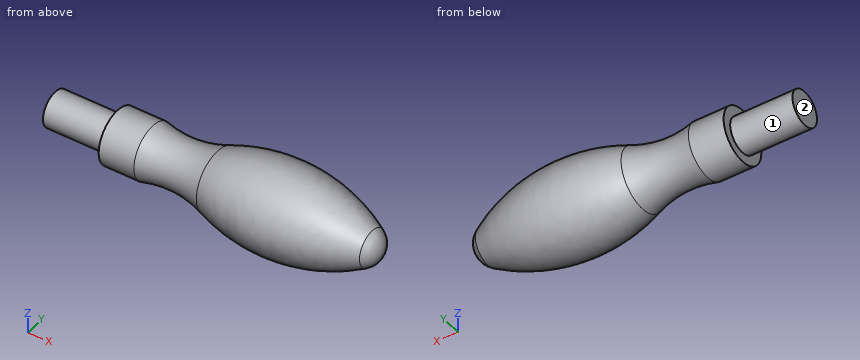
from build123d import *


with BuildPart() as f1:
    # F0 (on Front) → F1 (revolve)
    with BuildSketch(Plane.XZ):
        with BuildLine():
            Line((0, 6.5), (0, 0))
            Line((0, 0), (120.8, 0))
            ThreePointArc((120.8, 0), (119.780303, 3.855839), (116.987822, 6.703527))
            ThreePointArc((116.987822, 6.703527), (88.997191, 15.626515), (59.937706, 11.308939))
            ThreePointArc((59.937706, 11.308939), (48.07478, 8.717289), (36, 10))
            Line((36, 10), (23, 10))
            Line((23, 10), (23, 6.5))
            Line((23, 6.5), (0, 6.5))
        make_face()
    revolve(axis=Axis((60.4, 0, 0), (1, 0, 0)))


solid = f1.part
Read the model definition and answer for the solid it produces. Units are mm, in the model's axes. Face numbers are marked on the shaded views. A direction names the side the tool comes from. Coordinates: 2 decimals unless noted, no trailing zeros. Write each loop counter-clockwise with the first axis right and the second up, starting at its lowest first coordinate (ties: lowest second). Pieces come first, ordered by that corner, then holes. Notation, with made-up numbers: M 75.5,7.5 L 87.5,7.5 A19 ccw 87.5,30.5 Z; hole C -28,41 d2. An arc over 180 degrees is marked long. Use a Markdown table: item, result.
Q1. The part is cut by section A-A, the plane x = 29. Write down the section's boundary in (y, z).
Answer block:
| item | result |
|---|---|
| outline | C 0,0 d20 |
Q2. The part is cut by section B-B, the plane x = 42.5. Write down the section's boundary in (y, z), then the cut area to 3 significant figures.
Answer block:
| item | result |
|---|---|
| outline | C 0,0 d17.64 |
| area | 245 mm2 |
Q3. Which of the six approach directions +Z, -Z, +X, -X, +Y, -Y give full straight-line access (tool end or side, diameter ignored) to the marked faces 1 and 2?
Answer block:
| item | result |
|---|---|
| face 1 | -X |
| face 2 | +Z, -Z, -X, +Y, -Y |
Q4. Each of these flat-tipped pins is pushed along its axis until it touches: pin 1 Ø2 at (x, z) = (21, 4) entering from +Y; pin 2 Ø2 at (x, z) = (82.5, 5) entering from +Y; pin 3 Ø1 at (y, z) = (-8, 8.5) entering from +X. Where does it stop, or does it pass through?
Answer block:
| item | result |
|---|---|
| pin 1 | stops at y = 5.77 |
| pin 2 | stops at y = 15.31 |
| pin 3 | stops at x = 107.94 |
Q5. Straight lines are drawn through the part: L1, parallel to Z at x = 83, y = 0.5; L2, parallel to X at y = 6, z = -9.5; L3, parallel to Z at x = 33.5, y = -3. For each, find the intervals that lie inside material, in ascending order. Write a range as [from, to].
Answer block:
| item | result |
|---|---|
| L1 | z = [-15.82, 15.82] |
| L2 | x = [59.75, 107.78] |
| L3 | z = [-9.54, 9.54] |
